```python
from build123d import *
from build123d.topology import SkipClean

# Parameters (mm, degrees)
SKETCH1_R           = 6
BOSS_EXTRUDE1_DEPTH = 6
SKETCH2_R           = 3.5
BOSS_EXTRUDE2_DEPTH = 1
SKETCH4_R           = 1.65
CUT_EXTRUDE1_DEPTH  = 12
SKETCH6_R           = 6
SKETCH6_R_2         = 5
BOSS_EXTRUDE4_DEPTH = 0.6
FILLET3_R           = 3
BOSS_EXTRUDE5_DEPTH = 6
FILLET1_START       = 6
FILLET1_DEPTH       = 7
CUT_EXTRUDE2_DEPTH  = 3
SKETCH9_R           = 7.5
SKETCH9_R_2         = 6
BOSS_EXTRUDE6_DEPTH = 2.6


with BuildPart() as part:
    # Sketch1 → Boss-Extrude1 (new body)
    with BuildSketch(Plane.XY):
        with BuildLine():
            ThreePointArc((-0.145833333, -6.998480738), (7, 0), (-0.145833333, 6.998480738))
            Line((-0.145833333, 6.998480738), (-137.740421511, 4.131304533))
            ThreePointArc((-137.740421511, 4.131304533), (-151.5, 0), (-137.740421511, -4.131304533))
            Line((-137.740421511, -4.131304533), (-0.145833333, -6.998480738))
        make_face()
        with Locations((-144, 0)):
            Circle(SKETCH1_R, mode=Mode.SUBTRACT)
    extrude(amount=BOSS_EXTRUDE1_DEPTH)

    # Sketch2 → Boss-Extrude2 (add)
    with BuildSketch(Plane.XY.offset(6)):
        Circle(SKETCH2_R)
    extrude(amount=BOSS_EXTRUDE2_DEPTH)

    # Sketch4 → Cut-Extrude1 (cut)
    with BuildSketch(Plane.XY.offset(7)):
        Circle(SKETCH4_R)
    extrude(amount=-CUT_EXTRUDE1_DEPTH, mode=Mode.SUBTRACT)

    # Sketch6 → Boss-Extrude4 (add)
    with BuildSketch(Plane(origin=(0, 0, 0), x_dir=(-1, 0, 0), z_dir=(0, 0, -1))):
        with Locations((144, 0)):
            Circle(SKETCH6_R)
        with Locations((144, 0)):
            Circle(SKETCH6_R_2, mode=Mode.SUBTRACT)
    extrude(amount=-BOSS_EXTRUDE4_DEPTH)

    # Fillet3
    fillet3_edges = [part.edges().sort_by_distance(p)[0] for p in [
        (-137.740421511, -4.131304533, 3),
        (-137.740421511, 4.131304533, 3),
    ]]
    fillet(fillet3_edges, radius=FILLET3_R)

    # Sketch7 → Boss-Extrude5 (add)
    with SkipClean():  # the faces are left unmerged after this step: merging them gives an invalid solid
        with BuildSketch(Plane.XY.offset(6)):
            with BuildLine():
                ThreePointArc((-145.753823306, -5.737952929), (-149.088514051, 3.179154723), (-139.612167999, 4.092301349))
                Line((-139.612167999, 4.092301349), (-138.515209999, 5.115376687))
                ThreePointArc((-138.515209999, 5.115376687), (-150.360642563, 3.973943404), (-146.192279132, -7.172441161))
                Line((-146.192279132, -7.172441161), (-145.753823306, -5.737952929))
            make_face()
        extrude(amount=BOSS_EXTRUDE5_DEPTH)

    # Fillet1: read off the stored shape, not the designer's step
    # Fillet1 outline → Fillet1 (cut)
    with SkipClean():  # the faces are left unmerged after this step: merging them gives an invalid solid
        with BuildSketch(Plane.XY.offset(FILLET1_START)):
            with BuildLine():
                ThreePointArc((-145.753823306, -5.737952929), (-146.070376054, -5.631477869), (-146.380513939, -5.507554211))
                ThreePointArc((-146.380513939, -5.507554211), (-145.99732404, -5.881238582), (-145.960834066, -6.4152264))
                Line((-145.960834066, -6.4152264), (-145.753823306, -5.737952929))
            make_face()
            with BuildLine():
                Line((-146.192279132, -7.172441161), (-145.960834066, -6.4152264))
                ThreePointArc((-145.960834066, -6.4152264), (-146.363318277, -6.876752629), (-146.975642424, -6.884442763))
                ThreePointArc((-146.975642424, -6.884442763), (-146.587970068, -7.039347337), (-146.192279132, -7.172441161))
            make_face()
            with BuildLine():
                ThreePointArc((-139.094254686, 4.575332001), (-139.590167355, 4.373973779), (-140.094037649, 4.554498667))
                ThreePointArc((-140.094037649, 4.554498667), (-139.846668472, 4.330108223), (-139.612167999, 4.092301349))
                Line((-139.612167999, 4.092301349), (-139.094254686, 4.575332001))
            make_face()
            with BuildLine():
                ThreePointArc((-139.117547061, 5.693123334), (-138.855955133, 5.139436001), (-139.094254686, 4.575332001))
                Line((-139.094254686, 4.575332001), (-138.515209999, 5.115376687))
                ThreePointArc((-138.515209999, 5.115376687), (-138.80833559, 5.412635279), (-139.117547061, 5.693123334))
            make_face()
        extrude(amount=FILLET1_DEPTH, mode=Mode.SUBTRACT)

    # Sketch8 → Cut-Extrude2 (cut)
    with SkipClean():  # the faces are left unmerged after this step: merging them gives an invalid solid
        with BuildSketch(Plane.XY.offset(6)):
            with BuildLine():
                Line((-8.018864585, 3.833772393), (-106.262176435, 1.786592415))
                ThreePointArc((-106.262176435, 1.786592415), (-107.476577581, 1.260839283), (-107.975717263, 0.035259389))
                ThreePointArc((-107.975717263, 0.035259389), (-107.975700008, 0), (-107.975717263, -0.035259389))
                ThreePointArc((-107.975717263, -0.035259389), (-107.476577581, -1.260839283), (-106.262176435, -1.786592415))
                Line((-106.262176435, -1.786592415), (-8.018864585, -3.833772393))
                ThreePointArc((-8.018864585, -3.833772393), (-6.60867738, -3.168296566), (-6.289168562, -1.642059316))
                ThreePointArc((-6.289168562, -1.642059316), (-6.5, 0), (-6.289168562, 1.642059316))
                ThreePointArc((-6.289168562, 1.642059316), (-6.60867738, 3.168296566), (-8.018864585, 3.833772393))
            make_face()
        extrude(amount=-CUT_EXTRUDE2_DEPTH, mode=Mode.SUBTRACT)

    # Sketch9 → Boss-Extrude6 (add)
    with BuildSketch(Plane.XY.offset(6)):
        with Locations(Location((-144, 0, 0), (0, 0, 246.624693124))):
            Circle(SKETCH9_R)
        with Locations(Location((-144, 0, 0), (0, 0, 180))):
            Circle(SKETCH9_R_2, mode=Mode.SUBTRACT)
    extrude(amount=BOSS_EXTRUDE6_DEPTH)


solid = part.part
```
Geometry: final body of the model. Coordinates: model frame, mm. A direction names the side the tool comes from. Coordinates: 2 decimals unless noted, no trailing zeros. Order: outer loops, then holes, each group sorted by start corner. A loop starts at its lowest first (then second) coordinate and runs counter-clockwise, first axis right, second up. Notation, with made-up numbers: M -6,20 L 40,20 A27 cw 40,49 Z; hole C -16.75,-6.75 d8. An arc over 180 degrees is marked long. Answer in a Markdown table with one row per item. Add a question column.
Q1. Section query D-D on x = -34.5. Return the cut outline in (y, z), and give its area (3 significant figures).
Q2. Section query C-C on z = 10. Return the cut outline in (x, y), and give its area (3 significant figures).
Q3. Section query B-B on x = -95. Return the cut outline in (y, z).
Q4. Reachability of faces 1 (the cylindrical face through (-140, -3, 0.3)), 2 (the cylindrical face through (-6.5, 0, 4.5)), 3 (the flat face through (1, -2, 7)) from +Z, -Z, +X, -X, +Y, -Y: full face, straight path, thin tool, end or side. Return the list, or none.
Q5. Mould query, pull axis Y, two halves, no side actions, for faces 4 (the flat face through (-54, 0, 0)), 5 (the cylindrical face through (7, 0, 3)), 6 (the flat face through (-140, 4, 0.6)). Classes: released by +Y, released by -Y, zero draft, split by the parting line, or undercut.
Q6. Section query A-A on x = -144. Return the cut outline in (y, z).
Q7. Contact query for flat-ended pins moving along their axis: P1, Ø5, axis at x = -52.5, z = 6.5, coming from the -Y side; P2, Ø3, axis at x = -132.5, z = 6, coming from the +Y side; P3, Ø6, axis at y = 4.5, z = 10, coming from the -X side. Output: stop coordinate, or through.
Q8. Line query: L1, parallel to Y at x = -144, z = 0.2; L2, parallel to X at y = -1, z = 2.5; L3, parallel to Y at x = -144, z = 5. Output: solid intervals per line, ascending.
Completed:
| question | item | result |
|---|---|---|
| 1 | outline | M -6.28,0 L 6.28,0 L 6.28,6 L 3.28,6 L 3.28,3 L -3.28,3 L -3.28,6 L -6.28,6 Z |
| 1 | area | 55.7 mm2 |
| 2 | outline | M -146.98,-6.88 A0.75 ccw -146.38,-5.51 A6 cw long -140.09,4.55 A0.75 ccw -139.12,5.69 A7.5 ccw long Z |
| 2 | area | 36.6 mm2 |
| 3 | outline | M -5.02,0 L 5.02,0 L 5.02,6 L 2.02,6 L 2.02,3 L -2.02,3 L -2.02,6 L -5.02,6 Z |
| 4 | face 1 | +Z, -Z |
| 4 | face 2 | +Z |
| 4 | face 3 | +Z, +X, +Y, -Y |
| 5 | face 4 | zero draft |
| 5 | face 5 | split by the parting line |
| 5 | face 6 | undercut |
| 6 | outline | M -7.5,0 L -5,0 L -5,0.6 L -6,0.6 L -6,8.6 L -7.5,8.6 Z; M 5,0 L 7.5,0 L 7.5,12 L 6,12 L 6,0.6 L 5,0.6 Z |
| 7 | P1 | stops at y = -5.96 |
| 7 | P2 | stops at y = 4.27 |
| 7 | P3 | stops at x = -151.35 |
| 8 | L1 | y = -7.5 to -5, 5 to 7.5 |
| 8 | L2 | x = -151.43 to -149.92, -138.08 to -1.31, 1.31 to 6.93 |
| 8 | L3 | y = -7.5 to -6, 6 to 7.5 |
